Autodesk Inventor part; units mm, degrees
ref_plane "YZ Plane" through (0, 0, 0) normal (1, 0, 0) x (0, 1, 0)
ref_plane "XZ Plane" through (0, 0, 0) normal (0, 1, 0) x (-1, 0, 0)
ref_plane "XY Plane" through (0, 0, 0) normal (0, 0, 1) x (1, 0, 0)
sketch "Sketch1" plane through (0, 0, 0) normal (0, 1, 0) x (-1, 0, 0)
  line L0 (0, 0) -> (-5, 0)
  line L1 (-5, 0) -> (-5, 58)
  line L2 (-5, 58) -> (0, 58)
  line L3 (0, 58) -> (0, 0)
  line L4 (-5, 58) -> (-20, 58)
  line L5 (-20, 58) -> (-20, 53)
  line L6 (-20, 53) -> (-5, 53)
  line L7 (-5, 53) -> (-5, 58)
  line L8 (-5, 0) -> (-20, 0)
  line L9 (-20, 0) -> (-20, 5)
  line L10 (-20, 5) -> (-5, 5)
  line L11 (-5, 5) -> (-5, 0)
  point P0 (-5, 5)
  dimension "d0" = 5
  dimension "d1" = 5
  dimension "d2" = 5
  dimension "d3" = 15
  dimension "d4" = 15
  dimension "d5" = 48
extrude "Extrusion1" add sketch "Sketch1" along normal blind 20
sketch "Sketch2" plane through (0, 0, 58) normal (0, 0, 1) x (1, 0, 0)
  circle A0 centre (10, 10) radius 2.5
  line L0 (20, 0) -> (20, 20)
  line L1 (20, 0) -> (10, 0)
  line L2 (10, 0) -> (10, 20)
  line L3 (10, 20) -> (20, 20)
  line L4 (20, 20) -> (20, 0)
  line L5 (0, 0) -> (20, 0)
  line L6 (10, 4) -> (7, 4)
  line L7 (7, 4) -> (7, 16)
  line L8 (7, 16) -> (10, 16)
  line L9 (10, 16) -> (10, 4)
  dimension "d8" = 10
  dimension "d9" = 10
  dimension "d10" = 10
  dimension "d11" = 5
  dimension "d54" = 12
  dimension "d55" = 4
  dimension "d56" = 3
extrude "Extrusion2" cut sketch "Sketch2" against normal blind 200 contours A0 L2 | A0 L2 L3 L0 L1 | L2 A0
sketch "Sketch3" plane through (0, 0, 0) normal (-1, 0, 0) x (0, 0, 1)
  line L0 (5, 0) -> (5, 20)
  line L1 (53, 0) -> (53, 20)
  line L2 (5, 15) -> (53, 15)
  line L3 (53, 15) -> (53, 5)
  line L4 (53, 5) -> (5, 5)
  line L5 (5, 5) -> (5, 15)
  line L6 (0, 20) -> (58, 20)
  line L7 (0, 0) -> (58, 0)
  point P0 (5, 5)
  dimension "d14" = 5
  dimension "d15" = 5
extrude "Extrusion3" cut sketch "Sketch3" against normal blind 20 contours L0 L2 L1 L4
sketch "Sketch4" plane through (0, 0, 0) normal (-1, 0, 0) x (0, 0, 1)
  line L0 (58, 0) -> (58, 20)
  line L1 (58, 20) -> (68, 20)
  line L2 (68, 20) -> (68, 0)
  line L3 (68, 0) -> (58, 0)
  line L4 (58, 0) -> (58, 20)
  line L5 (20, 20) -> (10.5196, 12.6519)
  line L6 (20, 20) -> (10, 20)
  line L7 (10, 20) -> (10, 0)
  line L8 (10, 0) -> (20, 0)
  line L9 (20, 0) -> (20, 20)
  circle A0 centre (63, 3) radius 1.375
  circle A1 centre (63, 17) radius 1.375
  circle A2 centre (15, 17) radius 1.375
  circle A3 centre (15, 3) radius 1.375
  line L10 (0, 0) -> (58, 0)
  line L11 (0, 20) -> (58, 20)
  line L12 (0, 0) -> (0, 20)
  point P0 (10.5196, 0.1519)
  point P1 (63, 20)
  dimension "d18" = 10
  dimension "d19" = 10
  dimension "d20" = 3
  dimension "d21" = 3
  dimension "d22" = 5
  dimension "d23" = 5
  dimension "d24" = 5
  dimension "d25" = 5
  dimension "d26" = 3
  dimension "d27" = 3
  dimension "d28" = 2.75
  dimension "d29" = 2.75
  dimension "d30" = 2.75
  dimension "d31" = 2.75
  dimension "d63" = 0
  dimension "d64" = 0
  dimension "d65" = 10
extrude "Extrusion4" add sketch "Sketch4" against normal blind 5 contours L0 L1 L2 L3 | L8 L7 L6 L9
sketch "Sketch5" plane through (10, 12.5, 58) normal (1, 0, 0) x (0, 0, -1)
  circle A0 centre (55.5, 5) radius 1.375
  circle A1 centre (55.5, -10) radius 1.375
  circle A2 centre (2.5, 5) radius 1.375
  circle A3 centre (2.5, -10) radius 1.375
  line L0 (53, 7.5) -> (58, 7.5)
  line L1 (58, 7.5) -> (58, 0)
  line L2 (58, -5) -> (58, -12.5)
  line L3 (58, -12.5) -> (53, -12.5)
  line L4 (5, -12.5) -> (0, -12.5)
  line L5 (0, -12.5) -> (0, -5)
  line L6 (0, 0) -> (0, 7.5)
  line L7 (0, 7.5) -> (5, 7.5)
  dimension "d34" = 2.5
  dimension "d35" = 2.5
  dimension "d36" = 2.5
  dimension "d37" = 2.5
  dimension "d38" = 2.5
  dimension "d39" = 2.5
  dimension "d40" = 2.5
  dimension "d41" = 2.5
  dimension "d42" = 2.75
  dimension "d43" = 2.75
  dimension "d44" = 2.75
  dimension "d45" = 2.75
extrude "Extrusion5" cut sketch "Sketch5" against normal blind 15
sketch "Sketch6" plane through (0, 0, 68) normal (-1, 0, 0) x (0, 0, 1)
  circle A0 centre (-12.5, 17.5) radius 1.375
  circle A1 centre (-12.5, 17.5) radius 2
  circle A2 centre (-12.5, 2.5) radius 1.375
  circle A3 centre (-12.5, 2.5) radius 2
  circle A4 centre (-65.5, 2.5) radius 1.375
  circle A5 centre (-65.5, 2.5) radius 2
  circle A6 centre (-65.5, 17.5) radius 1.375
  circle A7 centre (-65.5, 17.5) radius 2
  point P0 (-68, 0)
  dimension "d48" = 4
  dimension "d49" = 4
  dimension "d50" = 4
  dimension "d51" = 4
extrude "Extrusion6" cut sketch "Sketch6" against normal blind 3 contours A0 | A1 | A2 | A3 | A4 | A5 | A6 | A7
sketch "Sketch7" plane through (10, 10, 58) normal (0, 0, 1) x (1, 0, 0)
  line L0 (-10, -10) -> (-5, -10)
  line L1 (-5, -10) -> (-2, -10)
  line L2 (-2, -10) -> (-2, -5)
  line L3 (-2, -5) -> (-5, -5)
  line L4 (-5, -5) -> (-5, -10)
  line L5 (-5, 5) -> (-5, 10)
  line L6 (-5, 10) -> (-2, 10)
  line L7 (-2, 10) -> (-2, 5)
  line L8 (-2, 5) -> (-5, 5)
  line L9 (-5, 5) -> (-5, 10)
  line L10 (-5, 10) -> (-5, -10)
  line L11 (-5, -10) -> (0, -10)
  line L12 (0, -10) -> (0, -2.5)
  arc A0 (0, 2.5) -> (0, -2.5) centre (0, 0) ccw
  line L13 (0, 2.5) -> (0, 10)
  line L14 (-5, 10) -> (0, 10)
  point P0 (-2, 10)
  point P1 (-2, -10)
  dimension "d57" = 5
  dimension "d58" = 5
  dimension "d59" = 3
  dimension "d60" = 3
extrude "Extrusion7" cut sketch "Sketch7" against normal blind 1000 contours L2 L3 L10 L8 L7 L14 L13 A0 L12 L11
sketch "Sketch8" plane through (0, 0, 0) normal (-1, 0, 0) x (0, 0, 1)
  circle A0 centre (2.5, 17.5) radius 2
  circle A1 centre (55.5, 17.5) radius 2
  circle A2 centre (2.5, 2.5) radius 2
  circle A3 centre (55.5, 2.5) radius 2
  line L0 (10, 5) -> (5, 5)
  line L1 (5, 5) -> (5, 15)
  line L2 (5, 15) -> (10, 15)
  line L3 (10, 15) -> (10, 5)
  circle A4 centre (63, 17) radius 1.375
  circle A5 centre (63, 3) radius 1.375
  line L4 (0, 0) -> (68, 0)
  line L5 (68, 0) -> (68, 20)
  line L6 (0, 20) -> (68, 20)
  line L7 (0, 0) -> (0, 20)
  line L8 (20, 5) -> (20, 15)
  line L9 (20, 15) -> (53, 15)
  line L10 (53, 15) -> (53, 5)
  line L11 (53, 5) -> (20, 5)
extrude "Extrusion8" add sketch "Sketch8" against normal blind 5 contours L0 L1 L2 L3
sketch "Sketch9" plane through (0, 0, 0) normal (-1, 0, 0) x (0, 0, 1)
  circle A0 centre (15, 17) radius 1.375
  circle A1 centre (15, 3) radius 1.375
  line L0 (68, 0) -> (68, 20)
  circle A2 centre (63, 3) radius 1.375
  line L1 (0, 0) -> (68, 0)
  line L2 (0, 20) -> (68, 20)
  line L3 (20, 5) -> (20, 15)
  dimension "d68" = 5
  dimension "d69" = 3
  dimension "d70" = 3
  dimension "d71" = 3
  dimension "d72" = 5
  dimension "d73" = 5
  dimension "d74" = 2.75
  dimension "d75" = 2.75
  dimension "d76" = 2.75
extrude "Extrusion9" cut sketch "Sketch9" against normal blind 5 contours A0 | A1
sketch "Sketch10" plane through (0, 0, 0) normal (-1, 0, 0) x (0, 0, 1)
  line L0 (53, 5) -> (20, 5)
  line L1 (20, 5) -> (15, 5)
  line L2 (15, 5) -> (15, 15)
  line L3 (15, 15) -> (20, 15)
  line L4 (20, 15) -> (20, 5)
  point P0 (0, 0)
  dimension "d79" = 5
extrude "Extrusion10" cut sketch "Sketch10" against normal blind 5
sketch "Sketch11" plane through (5, 0, 0) normal (1, 0, 0) x (0, 0, -1)
  circle A0 centre (-63, 17) radius 1.375
  circle A1 centre (-63, 17) radius 2
  circle A2 centre (-63, 3) radius 1.375
  circle A3 centre (-63, 3) radius 2
  circle A4 centre (-15, 3) radius 1.375
  circle A5 centre (-15, 3) radius 2
  circle A6 centre (-15, 17) radius 1.375
  circle A7 centre (-15, 17) radius 2
  point P0 (0, 0)
  dimension "d82" = 4
  dimension "d83" = 4
  dimension "d84" = 4
  dimension "d85" = 4
extrude "Extrusion11" cut sketch "Sketch11" against normal blind 2 contours A0 | A1 | A2 | A3 | A4 | A5 | A6 | A7
equation "\"d14\" = d15"
equation "\"d19\" = d18"
equation "\"d20\" = d21"
equation "\"d24\" = d23"
equation "\"d25\" = d22"
equation "\"d26\" = d20"
equation "\"d27\" = d21"
equation "\"d34\" = d35"
equation "\"d37\" = d34"
equation "\"d38\" = d34"
equation "\"d39\" = d36"
equation "\"d40\" = d39"
equation "\"d41\" = d34"
equation "\"d44\" = d42"
equation "\"d45\" = d43"
equation "\"d49\" = d48"
equation "\"d50\" = d49"
equation "\"d51\" = d48"
equation "\"d75\" = d74"
equation "\"d76\" = d75"
properties part number "MotorDifferentialMountingBracket"
Check sheet for the modelled part. Datum: model origin and axes. Units: mm. A direction names the side the tool comes from. Round coordinates to 2 decimals unless told otherwise and drop trailing zeros. Order: outer loops, then holes, each group sorted by start corner. A loop starts at its lowest first (then second) coordinate and runs counter-clockwise, first axis right, second up.
1) Section check D-D (y = 14). Record the boundary of the cut face in (x, z), and give its area (3 significant figures).
2) Scan lines: line 1 (Y direction, x = 3.4, z = 63); line 2 (Z direction, x = 1, y = 8.25); line 3 (Y direction, x = 1.2, z = 63) (3 decimals). Record each from-to range of solid material in increasing order.
3) Section check C-C (x = 1.5). Give the number of separate pieces and of enclosed holes in the cut face, and give its area (3 significant figures).
4) Tool access check on faces 4 (the flat face through (3, 10, 53)), 5 (the cylindrical face through (1.479, 19.483, 55.24)), 6 (the flat face through (7, 17, 53)). Record the directions out of +Z, -Z, +X, -X, +Y, -Y that give a thin tool (end or side, any length) a straight path to the whole face; none if there is none.
5) Section check A-A (z = 21.5). Record the boundary of the cut face in (x, y).
6) Go/stop test with flat-tipped pins: pin 1 Ø0.9 at (x, y) = (6, 16.5) entering from +Z; pin 2 Ø3.5 at (y, z) = (2.5, 55.5) entering from -X; pin 3 Ø1 at (x, y) = (5, 9.5) entering from -Z; pin 4 Ø1.2 at (y, z) = (3.5, 14) entering from +X. Record where each tip stops, or that it passes through.
7) Section check B-B (z = 63). Record the boundary of the cut face in (x, y) (3 decimals).
8) Mould release check, pull along Z, two halves, no side actions. Record for faces 1 (the flat face through (7, 2, 58)), 2 (the cylindrical face through (5.535, 18.863, 2.679)), 3 (the flat face through (3, 0, 34)): +Z half, -Z half, draft (parallel to the pull), parting line (faces both ways), or undercut.
Result:
1. outline: (0, 0) - (5, 0) - (5, 15) - (0, 15) - close; (0, 53) - (5, 53) - (5, 68) - (0, 68) - close
1. area: 150 mm2
2. line 1: y = 0 to 1, 5 to 15, 19 to 20
2. line 2: z = 0 to 15, 53 to 68
2. line 3: y = 0 to 1.625, 4.375 to 15.625, 18.375 to 20
3. separate pieces: 1
3. enclosed holes: 9
3. area: 906 mm2
4. face 4: +X, -X
4. face 5: -X
4. face 6: +X, +Y, -Y
5. outline: (0, 0) - (5, 0) - (5, 5) - (0, 5) - close; (0, 15) - (5, 15) - (5, 20) - (0, 20) - close
6. pin 1: stops at z = 58
6. pin 2: stops at x = 3
6. pin 3: stops at z = 0
6. pin 4: stops at x = 3
7. outline: (0, 0) - (5, 0) - (5, 1) - (3, 1) - (3, 1.625) - (0, 1.625) - close; (0, 4.375) - (3, 4.375) - (3, 5) - (5, 5) - (5, 15) - (3, 15) - (3, 15.625) - (0, 15.625) - close; (0, 18.375) - (3, 18.375) - (3, 19) - (5, 19) - (5, 20) - (0, 20) - close
8. face 1: +Z half
8. face 2: undercut
8. face 3: draft
